```python
from build123d import *

# Parameters (mm, degrees)
SALIENTE_EXTRUIR1_DEPTH = 5


with BuildPart() as part:
    # Croquis1 → Saliente-Extruir1 (new body)
    with BuildSketch(Plane.XY):
        with BuildLine():
            Line((-64, 25.6), (-73.471195353, 25.6))
            Line((-73.471195353, 25.6), (-73.471195353, -7.284781413))
            Line((-73.471195353, -7.284781413), (-64, -7.284781413))
            Line((-64, -7.284781413), (-64, 4.23055831))
            ThreePointArc((-64, 4.23055831), (-64.711403332, 5.506534523), (-66.170820393, 5.572199097))
            Line((-66.170820393, 5.572199097), (-67.658359214, 4.828429687))
            ThreePointArc((-67.658359214, 4.828429687), (-69.788596668, 2.881633081), (-69, 5.657609293))
            Line((-69, 5.657609293), (-69, 12.657609293))
            ThreePointArc((-69, 12.657609293), (-69.788596668, 15.433585506), (-67.658359214, 13.4867889))
            Line((-67.658359214, 13.4867889), (-66.170820393, 12.74301949))
            ThreePointArc((-66.170820393, 12.74301949), (-64.711403332, 12.808684064), (-64, 14.084660276))
            Line((-64, 14.084660276), (-64, 25.6))
        make_face()
    extrude(amount=-SALIENTE_EXTRUIR1_DEPTH)


solid = part.part
```
Verification items for the finished model (mm, model axes). A direction names the side the tool comes from. Round coordinates to 2 decimals unless told otherwise and drop trailing zeros. Write each loop counter-clockwise with the first axis right and the second up, starting at its lowest first coordinate (ties: lowest second). Pieces come first, ordered by that corner, then holes. Notation, with made-up numbers: (36, 75) - (77, 75) arc R31 ccw to (77, 109) - close; hole circle Ø6 at (34.25, 66). An arc over 180 degrees is marked (long way). Answer as a JSON object with one key per item and string values. Group by question number.
Q1. Section check C-C, the plane x = -66.75. Enter the section's corners in (y, z), plus the area to 3 significant figures.
Q2. Go/stop test with flat-tipped pins: pin 1 Ø1.5 at (y, z) = (8, -3.5) entering from +X; pin 2 Ø4 at (x, y) = (-68.5, 20) entering from +Z; pin 3 Ø1 at (y, z) = (13, -1.5) entering from +X. Record where each tip stops, or that it passes through.
Q3. Tool access check on faces 5 (the cylindrical face through (-64.7, 5.5, -2.5)), 6 (the flat face through (-69, 25.6, -2)). Record the directions out of +Z, -Z, +X, -X, +Y, -Y that give a thin tool (end or side, any length) a straight path to the whole face; none if there is none.
Q4. Mould release check, pull along X, two halves, no side actions. Record for faces 1 (the flat face through (-73.471, 9, -2)), 2 (the flat face through (-69, -7.285, -2)), 3 (the cylindrical face through (-69.742, 2.854, -2.465)), 4 (the cylindrical face through (-64.73, 12.798, -2.465)): released by +X, released by -X, zero draft, split by the parting line, or undercut.
Q5. Thickness scan on line 1 (X direction, y = 5, z = -2.2); line 2 (Y direction, x = -69.5, z = -3.8); line 3 (X direction, y = 11, z = -1.5). Record the ranges inside material, lowest first.
Q6. Section check A-A, the plane x = -65.5. Enter the section's corners in (y, z).
Q7. Section check B-B, the plane z = -4.3. Enter the section's corners in (x, y).
Q8. Section check D-D, the plane y = 7.5. Enter the section's corners in (x, z).
Found:
{
 "1": {"outline": "(-7.28, -5) - (5.28, -5) - (5.28, 0) - (-7.28, 0) - close; (13.03, -5) - (25.6, -5) - (25.6, 0) - (13.03, 0) - close", "area": "126 mm^2"},
 "2": {"pin 1": "stops at x = -69", "pin 2": "stops at z = 0", "pin 3": "stops at x = -64.12"},
 "3": {"face 5": "+Z, -Z", "face 6": "+Z, -Z, +X, -X, +Y"},
 "4": {"face 1": "released by -X", "face 2": "zero draft", "face 3": "undercut", "face 4": "undercut"},
 "5": {"line 1": "x = -73.47 to -70.24, -67.32 to -64.21", "line 2": "y = -7.28 to 2.74, 5.57 to 12.74, 15.57 to 25.6", "line 3": "x = -73.47 to -69"},
 "6": {"outline": "(-7.28, -5) - (5.73, -5) - (5.73, 0) - (-7.28, 0) - close; (12.58, -5) - (25.6, -5) - (25.6, 0) - (12.58, 0) - close"},
 "7": {"outline": "(-73.47, -7.28) - (-64, -7.28) - (-64, 4.23) arc R1.5 ccw to (-66.17, 5.57) - (-67.66, 4.83) arc R1.5 cw (long way) to (-69, 5.66) - (-69, 12.66) arc R1.5 cw (long way) to (-67.66, 13.49) - (-66.17, 12.74) arc R1.5 ccw to (-64, 14.08) - (-64, 25.6) - (-73.47, 25.6) - close"},
 "8": {"outline": "(-73.47, -5) - (-69, -5) - (-69, 0) - (-73.47, 0) - close"}
}
